Source: CAD feature listing. Evaluate the final solid. Frame: model axes, mm. A direction names the side the tool comes from. Coordinates: 2 decimals unless noted, no trailing zeros. Loops run counter-clockwise (first coordinate to the right, second up) from the corner with the lowest first, then second, coordinate; pieces in that order, holes last. Notation, with made-up numbers: (58.5, 50.25) -> (96.5, 50.25) arc R11 cw to (96.5, 61.25) -> close; hole circle Ø5 at (-26.5, -21). An arc over 180 degrees is marked (long way). Answer as a JSON object with one key per item and string values. Group by question number.
from build123d import *

# Parameters (mm, degrees)
SKETCH1_R           = 41.1
SKETCH1_R_2         = 2
SKETCH1_R_3         = 2.5
BOSS_EXTRUDE2_DEPTH = 4.064
FILLET1_R           = 4
FILLET2_R           = 10


with BuildPart() as part:
    # Sketch1 → Boss-Extrude2 (new body)
    with BuildSketch(Plane(origin=(0, 0, 0), x_dir=(1, 0, 0), z_dir=(0, 1, 0))):
        with BuildLine():
            Line((-16, 46.419931064), (-16, 61.6))
            Line((-16, 61.6), (16, 61.6))
            Line((16, 61.6), (16, 46.419931064))
            ThreePointArc((16, 46.419931064), (0, -49.1), (-16, 46.419931064))
        make_face()
        with Locations(Location((0, 0, 0), (0, 0, 270))):
            Circle(SKETCH1_R, mode=Mode.SUBTRACT)
        with Locations(Location((-11.64685703, 43.466662183, 0), (0, 0, 270))):
            Circle(SKETCH1_R_2, mode=Mode.SUBTRACT)
        with Locations(Location((31.819805153, 31.819805153, 0), (0, 0, 270))):
            Circle(SKETCH1_R_2, mode=Mode.SUBTRACT)
        with Locations(Location((43.466662183, -11.64685703, 0), (0, 0, 270))):
            Circle(SKETCH1_R_2, mode=Mode.SUBTRACT)
        with Locations(Location((11.64685703, -43.466662183, 0), (0, 0, 270))):
            Circle(SKETCH1_R_2, mode=Mode.SUBTRACT)
        with Locations(Location((-31.819805153, -31.819805153, 0), (0, 0, 270))):
            Circle(SKETCH1_R_2, mode=Mode.SUBTRACT)
        with Locations(Location((-43.466662183, 11.64685703, 0), (0, 0, 270))):
            Circle(SKETCH1_R_2, mode=Mode.SUBTRACT)
        with Locations(Location((-8, 55.6, 0), (0, 0, 270))):
            Circle(SKETCH1_R_3, mode=Mode.SUBTRACT)
        with Locations(Location((8, 55.6, 0), (0, 0, 270))):
            Circle(SKETCH1_R_3, mode=Mode.SUBTRACT)
    extrude(amount=BOSS_EXTRUDE2_DEPTH)

    # Fillet1
    fillet1_edges = [part.edges().sort_by_distance(p)[0] for p in [
        (-16, 2.032, -61.6),
        (16, 2.032, -61.6),
    ]]
    fillet(fillet1_edges, radius=FILLET1_R)

    # Fillet2
    fillet2_edges = [part.edges().sort_by_distance(p)[0] for p in [
        (16, 2.032, -46.419931064),
        (-16, 2.032, -46.419931064),
    ]]
    fillet(fillet2_edges, radius=FILLET2_R)


solid = part.part
1. Section query C-C on y = 2.2. State how many separate pieces and enclosed holes the cut face has, then the cut area to 3 significant figures.
2. Reachability of faces 1 (the face through (0, 2, -61.6)), 2 (the face through (-16, 2, -55)), 3 (the face through (16, 2, -55)) from +Z, -Z, +X, -X, +Y, -Y: full face, straight path, thin tool, end or side. Return the list, or none.
3. Mould query, pull axis Z, two halves, no side actions, for faces 4 (the face through (-22, 4.064, -35)), 5 (the face through (-14.859, 2.06, -60.397)), 6 (the face through (-11.559, 2.004, -45.465)), 7 (the face through (-42.115, 2.004, -13.121)). Classes: pulls with the +Z half, pulls with the -Z half, needs draft (parallel to the pull), parting line crosses it, or undercut.
4. Section query A-A on z = 0. Return loops of the section in (x, y).
5. Section query B-B on x = -26.5. Return loops of the section in (y, z), then the cut area to 3 significant figures.
6. Pin query (flat end, axial travel): pin 1 Ø2 at (x, y) = (35.5, 3) entering from +Z; pin 2 Ø1.2 at (y, z) = (1.5, -55) entering from -X. Return the tip coordinate at first contact, or that it passes through.
7. Section query D-D on z = -54.5. Return loops of the section in (x, y) (3 decimals), then the cut area to 3 significant figures.
8. Ray query, L1, parallel to X at y = 2.4, z = -55.6; L2, parallel to X at y = 0.55, z = -12.5; L3, parallel to Z at x = -33, y = 2. Return the intervals inside material, ascending.
Solved:
{
 "1": {"separate pieces": "1", "enclosed holes": "9", "area": "2,590 mm^2"},
 "2": {"face 1": "-Z, +X, -X, +Y, -Y", "face 2": "-Z, -X, +Y, -Y", "face 3": "-Z, +X, +Y, -Y"},
 "3": {"face 4": "needs draft", "face 5": "pulls with the -Z half", "face 6": "undercut", "face 7": "undercut"},
 "4": {"outline": "(-49.1, 0) -> (-41.1, 0) -> (-41.1, 4.06) -> (-49.1, 4.06) -> close; (41.1, 0) -> (49.1, 0) -> (49.1, 4.06) -> (41.1, 4.06) -> close"},
 "5": {"outline": "(0, -41.33) -> (4.06, -41.33) -> (4.06, -31.42) -> (0, -31.42) -> close; (0, 31.42) -> (4.06, 31.42) -> (4.06, 41.33) -> (0, 41.33) -> close", "area": "80.6 mm^2"},
 "6": {"pin 1": "z = 34.94", "pin 2": "x = -16"},
 "7": {"outline": "(-16, 0) -> (-10.245, 0) -> (-10.245, 4.064) -> (-16, 4.064) -> close; (-5.755, 0) -> (5.755, 0) -> (5.755, 4.064) -> (-5.755, 4.064) -> close; (10.245, 0) -> (16, 0) -> (16, 4.064) -> (10.245, 4.064) -> close", "area": "93.6 mm^2"},
 "8": {"L1": "-16 to -10.5, -5.5 to 5.5, 10.5 to 16", "L2": "-47.48 to -45.28, -41.66 to -39.15, 39.15 to 47.48", "L3": "-36.36 to -24.5, 24.5 to 30.21, 33.43 to 36.36"}
}
